Design review of the part built by this model. Coordinates are the model's own, in mm. A direction names the side the tool comes from. Give positions to 0.01 mm unless a question says otherwise; leave off trailing zeros. Loops run counter-clockwise (first coordinate to the right, second up) from the corner with the lowest first, then second, coordinate; pieces in that order, holes last.
from build123d import *

# Parameters (mm, degrees)
F1_DEPTH = 4.064
F4_DEPTH = 5.842
F6_DEPTH = 5.842
F7_R     = 1.27


with BuildPart() as f1:
    # F0 (on Top) → F1 (new body)
    with BuildSketch(Plane.XY):
        with BuildLine():
            Line((-41.15909, -99.06), (82.03091, -99.06))
            Line((82.03091, -99.06), (82.03091, -93.218))
            Line((82.03091, -93.218), (-34.80909, -93.218))
            ThreePointArc((-34.80909, -93.218), (-38.760403, -91.581313), (-40.39709, -87.63))
            Line((-40.39709, -87.63), (-40.39709, 87.63))
            ThreePointArc((-40.39709, 87.63), (-38.760403, 91.581313), (-34.80909, 93.218))
            Line((-34.80909, 93.218), (82.03091, 93.218))
            Line((82.03091, 93.218), (82.03091, 99.06))
            Line((82.03091, 99.06), (-41.15909, 99.06))
            ThreePointArc((-41.15909, 99.06), (-44.751192, 97.572102), (-46.23909, 93.98))
            Line((-46.23909, 93.98), (-46.23909, -93.98))
            ThreePointArc((-46.23909, -93.98), (-44.751192, -97.572102), (-41.15909, -99.06))
        make_face()
    extrude(amount=-F1_DEPTH)

    # F3 (on face) → F4 (join, through all)
    with BuildSketch(Plane(origin=(0, 99.06, 0), x_dir=(-1, 0, 0), z_dir=(0, 1, 0))):
        Polygon((29.633703, -4.064), (-82.03091, -4.064), (-82.03091, -9.4488), align=None)
    extrude(amount=-F4_DEPTH)

    # F5 (on face) → F6 (join)
    with BuildSketch(Plane(origin=(0, -93.218, 0), x_dir=(-1, 0, 0), z_dir=(0, 1, 0))):
        Polygon((34.80909, 0), (-82.03091, 0), (-82.03091, -9.4488), (34.80909, -4.064), align=None)
    extrude(amount=-F6_DEPTH)

    # F7
    f7_edges = [f1.edges().sort_by_distance(p)[0] for p in [
        (23.61091, 93.218, 0),
    ]]
    fillet(f7_edges, radius=F7_R)


solid = f1.part
Q1. Insertion check: pin 1 (1.4 mm diameter, centred on y = 12.5, z = -2.5, fed in from +X); pin 2 (13.5 mm diameter, centred on x = -36, y = 34, fed in from -Z). Each pin has a flat end and moves straight along its axis. Give the tip position at first contact, or say it passes through.
Results:
pin 1: stops at x = -40.4
pin 2: stops at z = -4.06
Q2. Take a section at B-B (x = -7.5). Give the boundary of the cut face in (y, z).
Results:
outline: (-99.06, -5.32) - (-93.22, -5.32) - (-93.22, -1.27) arc R1.27 ccw to (-94.49, 0) - (-99.06, 0) - close; (93.22, -5.13) - (99.06, -5.13) - (99.06, 0) - (94.49, 0) arc R1.27 ccw to (93.22, -1.27) - close
Q3. Take a section at A-A (z = -5.75). Give the boundary of the cut face in (x, y), plus the area to 3 significant figures.
Results:
outline: (1.77, -99.06) - (82.03, -99.06) - (82.03, -93.22) - (1.77, -93.22) - close; (5.33, 93.22) - (82.03, 93.22) - (82.03, 99.06) - (5.33, 99.06) - close
area: 917 mm2
Q4. Draft analysis for pull direction Y (two halves, no side actions). For faces 3 (the face through (-38.8, 91.54, -2.65)), 4 (the face through (35, 99.06, -4)), 5 (the face through (26.98, 96.18, -6.794)), 6 (the face through (-38.72, -91.62, -2.65)), state which applies: pulls with the +Y half, pulls with the -Y half, needs draft (parallel to the pull), parting line crosses it, or undercut.
Results:
face 3: undercut
face 4: pulls with the +Y half
face 5: needs draft
face 6: undercut
Q5. Take a section at C-C (x = 13). Give the boundary of the cut face in (y, z).
Results:
outline: (-99.06, -6.27) - (-93.22, -6.27) - (-93.22, -1.27) arc R1.27 ccw to (-94.49, 0) - (-99.06, 0) - close; (93.22, -6.12) - (99.06, -6.12) - (99.06, 0) - (94.49, 0) arc R1.27 ccw to (93.22, -1.27) - close
Q6. Tool access review of faces 1 (the face through (-44.711, 97.611, -2.004)), 2 (the face through (37, 93.218, -4)): name each direction out of +Z, -Z, +X, -X, +Y, -Y from which nothing blocks a thin tool from reaching the whole face with its end or side.
Results:
face 1: +Z, -Z, -X, +Y
face 2: +Z, -Z, +X
Q7. Wall thickness on line 1 (Y direction, x = 34, z = -3); line 2 (X direction, y = -1, z = -1.5); line 3 (Y direction, x = 62, z = -0.5): over which ranges is each line inside the solid? List them lowest first.
Results:
line 1: y = -99.06 to -93.22, 93.22 to 99.06
line 2: x = -46.24 to -40.4
line 3: y = -99.06 to -93.48, 93.48 to 99.06
Q8. Take a section at D-D (y = 64). Give the boundary of the cut face in (x, z).
Results:
outline: (-46.24, -4.06) - (-40.4, -4.06) - (-40.4, -1.27) arc R1.27 ccw to (-41.67, 0) - (-46.24, 0) - close
